from build123d import *

# Parameters (mm, degrees)
SKETCH_1_W                = 1400
SKETCH_1_H                = 55
EXTRUDE_1_DEPTH           = 110
CUT_EXTRUDE_START         = -10
CUT_EXTRUDE_1_OUTLINE_R   = 30
CUT_EXTRUDE_1_OUTLINE_R_2 = 2.5
CUT_EXTRUDE_1_DEPTH       = 10
CUT_EXTRUDE_START_2       = -3
SKETCH_4_W                = 52
SKETCH_4_H                = 107
CUT_EXTRUDE_2_DEPTH       = 1394
SKETCH_5_R                = 20
CUT_EXTRUDE_3_DEPTH       = 10
EXTRUDE_START             = -45
SKETCH_7_R                = 30
EXTRUDE_2_DEPTH           = 52
SKETCH_8_R                = 27
CUT_EXTRUDE_4_DEPTH       = 47
PATTERN_LINEAR_1_COUNT    = 10
PATTERN_LINEAR_1_PITCH    = 155


# Read off the part's stored shape, not the designer's step: Вырез-Вытянуть1
with BuildPart() as part:
    # Эскиз1 → Бобышка-Вытянуть1 (new body)
    with BuildSketch(Plane(origin=(0, 0, 0), x_dir=(1, 0, 0), z_dir=(0, 1, 0))):
        with Locations((-700, 27.5)):
            Rectangle(SKETCH_1_W, SKETCH_1_H)
    extrude(amount=EXTRUDE_1_DEPTH)

    # Вырез-Вытянуть1 outline → Вырез-Вытянуть1 (cut)
    with BuildSketch(Plane(origin=(0, 0, -55), x_dir=(-1, 0, 0), z_dir=(0, 0, -1)).offset(CUT_EXTRUDE_START)):
        with Locations((60, 55)):
            Circle(CUT_EXTRUDE_1_OUTLINE_R)
        with Locations((15, 95)):
            Circle(CUT_EXTRUDE_1_OUTLINE_R_2)
        with Locations((1300, 55)):
            Circle(CUT_EXTRUDE_1_OUTLINE_R)
        with Locations((1145, 55)):
            Circle(CUT_EXTRUDE_1_OUTLINE_R)
        with Locations((990, 55)):
            Circle(CUT_EXTRUDE_1_OUTLINE_R)
        with Locations((835, 55)):
            Circle(CUT_EXTRUDE_1_OUTLINE_R)
        with Locations((680, 55)):
            Circle(CUT_EXTRUDE_1_OUTLINE_R)
        with Locations((525, 55)):
            Circle(CUT_EXTRUDE_1_OUTLINE_R)
        with Locations((370, 55)):
            Circle(CUT_EXTRUDE_1_OUTLINE_R)
        with Locations((215, 55)):
            Circle(CUT_EXTRUDE_1_OUTLINE_R)
        with Locations((15, 15)):
            Circle(CUT_EXTRUDE_1_OUTLINE_R_2)
    extrude(amount=CUT_EXTRUDE_1_DEPTH, mode=Mode.SUBTRACT)

    # Эскиз4 → Вырез-Вытянуть2 (cut)
    with BuildSketch(Plane(origin=(0, 0, 0), x_dir=(0, 0, -1), z_dir=(1, 0, 0)).offset(CUT_EXTRUDE_START_2)):
        with Locations((27.5, 55)):
            Rectangle(SKETCH_4_W, SKETCH_4_H)
    extrude(amount=-CUT_EXTRUDE_2_DEPTH, mode=Mode.SUBTRACT)

    # Эскиз5 → Вырез-Вытянуть3 (cut)
    with BuildSketch(Plane.XY):
        with Locations((-1370, 55)):
            Circle(SKETCH_5_R)
    extrude(amount=-CUT_EXTRUDE_3_DEPTH, mode=Mode.SUBTRACT)

    # Эскиз7 → Бобышка-Вытянуть2 (add)
    with BuildSketch(Plane(origin=(0, 0, -55), x_dir=(-1, 0, 0), z_dir=(0, 0, -1)).offset(EXTRUDE_START)):
        with Locations((60, 55)):
            Circle(SKETCH_7_R)
    extrude_2 = extrude(amount=EXTRUDE_2_DEPTH)

    # Эскиз8 → Вырез-Вытянуть4 (cut)
    with BuildSketch(Plane(origin=(0, 0, -62), x_dir=(-1, 0, 0), z_dir=(0, 0, -1))):
        with Locations((60, 55)):
            Circle(SKETCH_8_R)
    cut_extrude_4 = extrude(amount=-CUT_EXTRUDE_4_DEPTH, mode=Mode.SUBTRACT)

    # Линейный массив1: Бобышка-Вытянуть2, Вырез-Вытянуть4 ×10, 1 skipped
    with Locations(*[(-i * PATTERN_LINEAR_1_PITCH, 0, 0) for i in range(1, PATTERN_LINEAR_1_COUNT) if i not in (9,)]):
        add(extrude_2)
        add(cut_extrude_4, mode=Mode.SUBTRACT)


solid = part.part
Source: CAD feature listing. Evaluate the final solid. Frame: model axes, mm. A direction names the side the tool comes from. Give positions to 0.01 mm unless a question says otherwise; leave off trailing zeros. Write each loop counter-clockwise with the first axis right and the second up, starting at its lowest first coordinate (ties: lowest second). Pieces come first, ordered by that corner, then holes. Notation, with made-up numbers: M -40,-35.75 L 7,-35.75 A27 ccw 7,1.25 Z; hole C 56,61 d4. An arc over 180 degrees is marked long. Return JSON: item names as keys, results as strings. Group by question number.
1) Draft query along X for faces 6 (the face through (-1275, 66, -62)), 7 (the face through (-383.843, 28.385, -58.451)). Return one class per face: released by +X, released by -X, zero draft, split by the parting line, or undercut.
2) Cut plane A-A, the plane z = -39.5. Give the number of separate pieces and of enclosed holes in the cut face, then the cut area to 3 significant figures.
3) Ray query, L1, parallel to Y at x = -680, z = -32; L2, parallel to Z at x = -713, y = 20; L3, parallel to Y at x = -15, z = -53.75. Return the intervals inside material, ascending.
4) Cut plane C-C, the plane x = -1043.5. Output: boundary loops of the cut face in (y, z).
5) Set-up query: faces 1 (the face through (-383.843, 28.385, -31.446)), 2 (the face through (-1351.525, 47.34, -0.74)), 3 (the face through (-710, 54, 0)), 4 (the face through (-655, 66, -62)), 5 (the face through (-704.94, 44.66, -38.83)). Return all of +Z, -Z, +X, -X, +Y, -Y with unobstructed straight access to the full face (end or side cutting, diameter ignored); none if empty.
6) First-contact query: pin 1 Ø15.5 at (x, z) = (-577.5, -25) entering from -Y; pin 2 Ø16 at (x, y) = (-369, 64.5) entering from -Z; pin 3 Ø4.5 at (x, y) = (-15, 95) entering from -Z; pin 4 Ø8 at (x, y) = (-669, 99) entering from -Z. Flat tips, straight axial feed; report the tip coordinate or a pass-through.
7) Cut plane B-B, the plane x = -525. Output: boundary loops of the cut face in (y, z).
Data:
{
 "1": {"face 6": "zero draft", "face 7": "undercut"},
 "2": {"separate pieces": "10", "enclosed holes": "10", "area": "9,680 mm²"},
 "3": {"L1": "y = 0 to 1.5, 25 to 28, 82 to 85, 108.5 to 110", "L2": "z = -55 to -53.5, -1.5 to 0", "L3": "y = 0 to 12.5, 17.5 to 92.5, 97.5 to 110"},
 "4": {"outline": "M 0,-55 L 110,-55 L 110,0 L 0,0 Z; hole M 1.5,-53.5 L 108.5,-53.5 L 108.5,-1.5 L 1.5,-1.5 Z"},
 "5": {"face 1": "none", "face 2": "+Z", "face 3": "+Z, +X, -X, +Y, -Y", "face 4": "-Z, +X, -X, +Y, -Y", "face 5": "-Z"},
 "6": {"pin 1": "stops at y = 0", "pin 2": "stops at z = -15", "pin 3": "stops at z = -1.5", "pin 4": "stops at z = -55"},
 "7": {"outline": "M 0,-55 L 25,-55 L 25,-62 L 28,-62 L 28,-15 L 82,-15 L 82,-62 L 85,-62 L 85,-55 L 110,-55 L 110,0 L 0,0 Z; hole M 1.5,-53.5 L 25,-53.5 L 25,-10 L 85,-10 L 85,-53.5 L 108.5,-53.5 L 108.5,-1.5 L 1.5,-1.5 Z"}
}
